```python
from build123d import *

# Parameters (mm, degrees)
CROQUIS2_R                   = 1.5
SALIENTE_EXTRUIR1_DEPTH      = 10
CORTAR_EXTRUIR_L_MINA2_START = -0.6
CORTAR_EXTRUIR_L_MINA2_DEPTH = 0.6


# Read off the part's stored shape, not the designer's step: Cortar-Extruir-Lámina2
with BuildPart() as part:
    # Croquis2 → Saliente-Extruir1 (new body)
    with BuildSketch(Plane.XY):
        Circle(CROQUIS2_R)
    extrude(amount=-SALIENTE_EXTRUIR1_DEPTH)

    # Croquis4 → Revolución1 (revolve)
    with BuildSketch(Plane(origin=(0, 0, 0), x_dir=(1, 0, 0), z_dir=(0, 1, 0))):
        with BuildLine():
            Line((2, 10), (0, 10))
            Line((0, 10), (0, 11.5))
            ThreePointArc((0, 11.5), (1.25, 11.083333333), (2, 10))
        make_face()
    revolve(axis=Axis((0, 0, -10), (0, 0, -1)))

    # Cortar-Extruir-Lámina2 outline → Cortar-Extruir-Lámina2 (cut)
    with BuildSketch(Plane(origin=(0, 0, -11.5), x_dir=(-1, 0, 0), z_dir=(0, 0, -1)).offset(CORTAR_EXTRUIR_L_MINA2_START)):
        Polygon((0.1, -1), (0.1, -0.1), (1, -0.1), (1, 0.1), (0.1, 0.1), (0.1, 1), (-0.1, 1), (-0.1, 0.1), (-1, 0.1), (-1, -0.1), (-0.1, -0.1), (-0.1, -1), align=None)
    extrude(amount=CORTAR_EXTRUIR_L_MINA2_DEPTH, mode=Mode.SUBTRACT)


solid = part.part
```
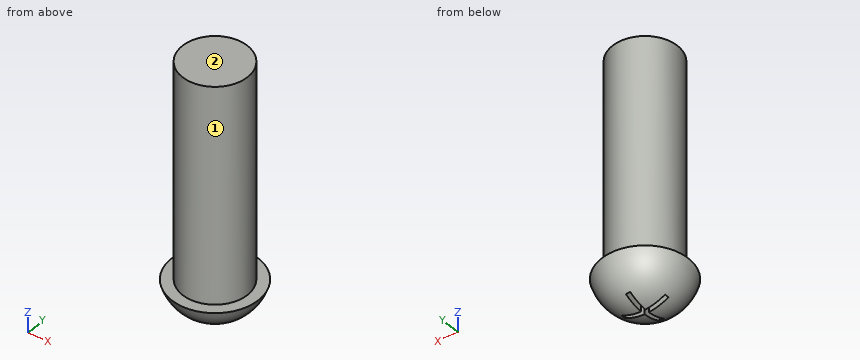
Could you check a few things on this model? Use its own coordinates, in mm. Face numbers are marked on the shaded views. A direction names the side the tool comes from. Round coordinates to 2 decimals unless told otherwise and drop trailing zeros. Loops run counter-clockwise (first coordinate to the right, second up) from the corner with the lowest first, then second, coordinate; pieces in that order, holes last. Notation, with made-up numbers: M 88,-33.5 L 130,-33.5 A18 ccw 130,-11.5 Z; hole C 20,58.25 d9. An arc over 180 degrees is marked long. Put each result on its own line as item: value.
Q1. Imagine slicing it at A-A (y = 1.25). Write out the boundary of the cut face in (x, z).
Check result:
outline: M -1.56,-10 A1.67 ccw 1.56,-10 L 0.83,-10 L 0.83,0 L -0.83,0 L -0.83,-10 Z
Q2. On a 3-axis mill with a long thin cutter (end or side, diameter ignored), from which of +Z, -Z, +X, -X, +Y, -Y can I reach the whole of each face in a straight line? I mean the marked faces 1 and 2. Say none if no direction works.
Check result:
face 1: +Z
face 2: +Z, +X, -X, +Y, -Y
Q3. Imagine slicing it at D-D (x = -1.3). Write out the boundary of the cut face in (y, z), then the cut area to 3 significant figures.
Check result:
outline: M -1.52,-10 A1.63 ccw 1.52,-10 L 0.75,-10 L 0.75,0 L -0.75,0 L -0.75,-10 Z
area: 17.3 mm2
Q4. I need wall thicknesses on probe 1 along Y at (x, z) = (0, -5.5); probe 2 along Z at (x, y) = (0.7, -0.45); probe 3 along Z at (x, y) = (-0.9, 0). Which ranges of each line are inside material? Lowest first, please.
Check result:
probe 1: -1.5 to 1.5
probe 2: -11.33 to 0
probe 3: -10.9 to 0
Q5. Imagine slicing it at B-B (z = -3). Write out the boundary of the cut face in (x, y), then the cut area to 3 significant figures.
Check result:
outline: C 0,0 d3
area: 7.07 mm2
Q6. Imagine slicing it at C-C (x = -0.35). Write out the boundary of the cut face in (y, z).
Check result:
outline: M -1.97,-10 A2.05 ccw -0.1,-11.47 L -0.1,-10.9 L 0.1,-10.9 L 0.1,-11.47 A2.05 ccw 1.97,-10 L 1.46,-10 L 1.46,0 L -1.46,0 L -1.46,-10 Z
Q7. For pin 1 (0.5 mm diameter, centred on y = 0.5, z = -11.5, fed in from +X); pin 2 (0.5 mm diameter, centred on x = -0.5, z = -11, fed in from +Y); pin 3 (1 mm diameter, centred on y = 0.5, z = -1.5, fed in from -X), each with a flat end and sliding along its axis, tell me the tip position at first contact or that it passes through.
Check result:
pin 1: x = 0.87
pin 2: y = 1.53
pin 3: x = -1.5
